from build123d import *

# Parameters (mm, degrees)
BASE_FLANGE1_DEPTH = 10
SKETCH6_R          = 1.984375
CUT_EXTRUDE1_DEPTH = 10
SKETCH7_R          = 1.984375
CUT_EXTRUDE2_DEPTH = 10


# Sheet-metal steps are written as plain solids
with BuildPart() as part:
    # Sketch1 → Base-Flange1 (new body)
    with BuildSketch(Plane(origin=(0, 0, 0), x_dir=(1, 0, 0), z_dir=(0, 1, 0))):
        with BuildLine():
            Line((0, 40), (0, 0.7366))
            ThreePointArc((0, 0.7366), (0.215745145, 0.215745145), (0.7366, 0))
            Line((0.7366, 0), (40, 0))
            Line((40, 0), (40, -0.7366))
            Line((40, -0.7366), (0.7366, -0.7366))
            ThreePointArc((0.7366, -0.7366), (-0.30510971, -0.30510971), (-0.7366, 0.7366))
            Line((-0.7366, 0.7366), (-0.7366, 40))
            Line((-0.7366, 40), (0, 40))
        make_face()
    extrude(amount=BASE_FLANGE1_DEPTH)

    # Sketch6 → Cut-Extrude1 (cut)
    with BuildSketch(Plane.XY.offset(0.7366)):
        with Locations((35, 5)):
            Circle(SKETCH6_R)
    extrude(amount=-CUT_EXTRUDE1_DEPTH, mode=Mode.SUBTRACT)

    # Sketch7 → Cut-Extrude2 (cut)
    with BuildSketch(Plane.ZY.offset(0.7366)):
        with Locations((-35, 5)):
            Circle(SKETCH7_R)
    extrude(amount=-CUT_EXTRUDE2_DEPTH, mode=Mode.SUBTRACT)


solid = part.part
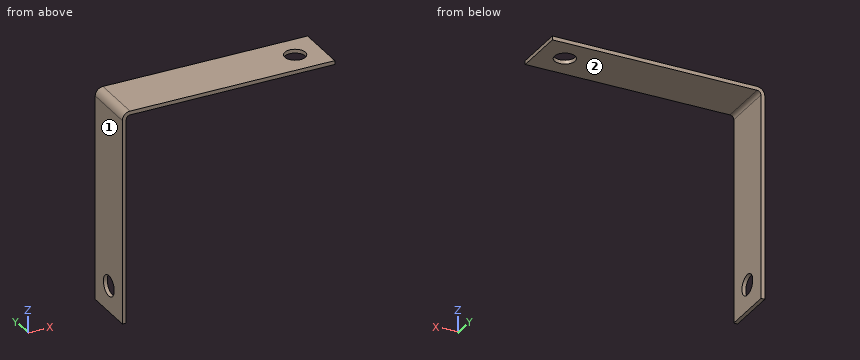
Model file for the job. Use its own axes, mm. Face numbers are marked on the shaded views. A direction names the side the tool comes from. Give positions to 0.01 mm unless a question says otherwise; leave off trailing zeros. Loops run counter-clockwise (first coordinate to the right, second up) from the corner with the lowest first, then second, coordinate; pieces in that order, holes last.
1) Flat gauge pins, fed straight in: pin 1 Ø3 at (y, z) = (5, -35) entering from -X; pin 2 Ø4.5 at (x, y) = (35, 5) entering from -Z. Where does each tip first touch, or does it go through?
2) Wall check: line 1 (X direction, y = 7, z = -27); line 2 (Z direction, x = 5.5, y = 5); line 3 (Y direction, x = 35, z = 0.3). Give the ranges that are in metal, low to high.
3) Saw through at C-C (z = -35). Write the cut outline in (x, y).
4) Saw through at D-D (y = 9.5). Write the cut outline in (x, z).
5) Saw through at A-A (y = 5). Write the cut outline in (x, z).
6) Tool access for the marked faces 1 and 2: list every direction of +Z, -Z, +X, -X, +Y, -Y with a clear straight run to the whole face (end or side of a thin tool).
7) Saw through at B-B (x = 35). Write the cut outline in (y, z), plus the area to 3 significant figures.
Answer block:
1. pin 1: passes through
1. pin 2: stops at z = 0
2. line 1: x = -0.74 to 0
2. line 2: z = 0 to 0.74
2. line 3: y = 0 to 3.02, 6.98 to 10
3. outline: (-0.74, 0) - (0, 0) - (0, 3.02) - (-0.74, 3.02) - close; (-0.74, 6.98) - (0, 6.98) - (0, 10) - (-0.74, 10) - close
4. outline: (-0.74, -40) - (0, -40) - (0, -0.74) arc R0.74 cw to (0.74, 0) - (40, 0) - (40, 0.74) - (0.74, 0.74) arc R1.47 ccw to (-0.74, -0.74) - close
5. outline: (-0.74, -40) - (0, -40) - (0, -36.98) - (-0.74, -36.98) - close; (-0.74, -33.02) - (0, -33.02) - (0, -0.74) arc R0.74 cw to (0.74, 0) - (33.02, 0) - (33.02, 0.74) - (0.74, 0.74) arc R1.47 ccw to (-0.74, -0.74) - close; (36.98, 0) - (40, 0) - (40, 0.74) - (36.98, 0.74) - close
6. face 1: +Z, -Z, -X, +Y, -Y
6. face 2: -Z, +X, +Y, -Y
7. outline: (0, 0) - (3.02, 0) - (3.02, 0.74) - (0, 0.74) - close; (6.98, 0) - (10, 0) - (10, 0.74) - (6.98, 0.74) - close
7. area: 4.44 mm2
